```python
from build123d import *

# Parameters (mm, degrees)
SKETCH4_W           = 110
SKETCH4_H           = 80
BOSS_EXTRUDE1_DEPTH = 20
SHELL1_T            = -5
FILLET1_R           = 5
SKETCH8_W           = 15
SKETCH8_H           = 15
CUT_EXTRUDE2_DEPTH  = 5
SKETCH10_R          = 2
SKETCH10_R_2        = 1
BOSS_EXTRUDE2_DEPTH = 15
FILLET2_R           = 1


with BuildPart() as part:
    # Sketch4 → Boss-Extrude1 (new body)
    with BuildSketch(Plane(origin=(0, 0, 0), x_dir=(1, 0, 0), z_dir=(0, 1, 0))):
        Rectangle(SKETCH4_W, SKETCH4_H)
    extrude(amount=BOSS_EXTRUDE1_DEPTH)

    # Shell1
    shell1_openings = [part.faces().sort_by_distance(p)[0] for p in [
        (0, 20, 0),
    ]]
    offset(amount=SHELL1_T, openings=shell1_openings, kind=Kind.INTERSECTION)

    # Fillet1
    fillet1_edges = [part.edges().sort_by_distance(p)[0] for p in [
        (55, 10, 40),
        (-55, 10, 40),
        (-55, 10, -40),
        (55, 10, -40),
    ]]
    fillet(fillet1_edges, radius=FILLET1_R)

    # Sketch8 → Cut-Extrude2 (cut)
    with BuildSketch(Plane.ZY.offset(55)):
        with Locations((0, 12.5)):
            Rectangle(SKETCH8_W, SKETCH8_H)
    extrude(amount=-CUT_EXTRUDE2_DEPTH, mode=Mode.SUBTRACT)

    # Sketch10 → Boss-Extrude2 (add)
    # profile 1 of 4: a face of its own
    with BuildSketch(Plane(origin=(0, 5, 0), x_dir=(1, 0, 0), z_dir=(0, 1, 0))):
        with Locations(Location((47.1, 31.5, 0), (0, 0, 90))):
            Circle(SKETCH10_R)
        with Locations(Location((47.1, 31.5, 0), (0, 0, 90))):
            Circle(SKETCH10_R_2, mode=Mode.SUBTRACT)
    # profile 2 of 4: a face of its own
    with BuildSketch(Plane(origin=(0, 5, 0), x_dir=(1, 0, 0), z_dir=(0, 1, 0))):
        with Locations(Location((47.1, -31.5, 0), (0, 0, 90))):
            Circle(SKETCH10_R)
        with Locations(Location((47.1, -31.5, 0), (0, 0, 90))):
            Circle(SKETCH10_R_2, mode=Mode.SUBTRACT)
    # profile 3 of 4: a face of its own
    with BuildSketch(Plane(origin=(0, 5, 0), x_dir=(1, 0, 0), z_dir=(0, 1, 0))):
        with Locations(Location((-46.5, 31.5, 0), (0, 0, 90))):
            Circle(SKETCH10_R)
        with Locations(Location((-46.412417336, 31.528728885, 0), (0, 0, 90))):
            Circle(SKETCH10_R_2, mode=Mode.SUBTRACT)
    # profile 4 of 4: a face of its own
    with BuildSketch(Plane(origin=(0, 5, 0), x_dir=(1, 0, 0), z_dir=(0, 1, 0))):
        with Locations(Location((-46.5, -31.5, 0), (0, 0, 90))):
            Circle(SKETCH10_R)
        with Locations(Location((-46.412417336, -31.528728885, 0), (0, 0, 90))):
            Circle(SKETCH10_R_2, mode=Mode.SUBTRACT)
    extrude(amount=BOSS_EXTRUDE2_DEPTH)

    # Fillet2
    fillet2_edges = [part.edges().sort_by_distance(p)[0] for p in [
        (-55, 0, 0),
        (55, 0, 0),
        (0, 0, 40),
        (0, 0, -40),
        (-53.535533906, 0, 38.535533906),
        (53.535533906, 0, 38.535533906),
        (53.535533906, 0, -38.535533906),
        (-53.535533906, 0, -38.535533906),
    ]]
    fillet(fillet2_edges, radius=FILLET2_R)


solid = part.part
```
Source: CAD feature listing. Evaluate the final solid. Frame: model axes, mm. A direction names the side the tool comes from. Coordinates: 2 decimals unless noted, no trailing zeros. Write each loop counter-clockwise with the first axis right and the second up, starting at its lowest first coordinate (ties: lowest second). Pieces come first, ordered by that corner, then holes. Notation, with made-up numbers: (33, 82) - (58, 82) arc R19 cw to (58, 98) - close; hole circle Ø7 at (70.25, 32). An arc over 180 degrees is marked (long way). Answer as a JSON object with one key per item and string values.
Q1. Draft query along X for faces 4 (the cylindrical face through (48.874, 12.395, -32.423)), 5 (the cylindrical face through (-54, 11, 38)), 6 (the flat face through (-53, 12, -7.5)). Return one class per face: released by +X, released by -X, zero draft, split by the parting line, or undercut.
Ans:
{"face 4": "undercut", "face 5": "released by -X", "face 6": "zero draft"}
Q2. First-contact query: pin 1 Ø4 at (x, z) = (-23.5, -23) entering from +Y; pin 2 Ø2.5 at (x, y) = (-51.5, 11) entering from +Z; pin 3 Ø2.5 at (x, y) = (-53, 12.5) entering from -Z. Flat tips, straight axial feed; report the tip coordinate or a pass-through.
Ans:
{"pin 1": "stops at y = 5", "pin 2": "stops at z = 39.99", "pin 3": "stops at z = -39.68"}
Q3. Section query B-B, the plane z = 10. Output: boundary loops of the cut face in (x, y).
Ans:
{"outline": "(-55, 1) arc R1 ccw to (-54, 0) - (54, 0) arc R1 ccw to (55, 1) - (55, 20) - (50, 20) - (50, 5) - (-50, 5) - (-50, 20) - (-55, 20) - close"}
Q4. Set-up query: faces 1 (the flat face through (-1, 10, -40)), 2 (the flat face through (-53, 12, 7.5)), 3 (the cylindrical face through (48.874, 12.395, 30.577)). Return all of +Z, -Z, +X, -X, +Y, -Y with unobstructed straight access to the full face (end or side cutting, diameter ignored); none if empty.
Ans:
{"face 1": "-Z, +X, -X, +Y, -Y", "face 2": "-X, +Y", "face 3": "+Y"}
Q5. Material intervals for line 1 (Z direction, x = 47.1, y = 8.75); line 2 (X direction, y = 12.5, z = 31.5); line 3 (X direction, y = 8.5, z = 10), sorted ascending. Write a range as [from, to].
Ans:
{"line 1": "z = [-40, -35], [-33.5, -32.5], [-30.5, -29.5], [29.5, 30.5], [32.5, 33.5], [35, 40]", "line 2": "x = [-55, -50], [-48.5, -47.41], [-45.41, -44.5], [45.1, 46.1], [48.1, 49.1], [50, 55]", "line 3": "x = [-55, -50], [50, 55]"}
Q6. Section query C-C, the plane x = -28. Output: boundary loops of the cut face in (y, z).
Ans:
{"outline": "(0, -39) arc R1 ccw to (1, -40) - (20, -40) - (20, -35) - (5, -35) - (5, 35) - (20, 35) - (20, 40) - (1, 40) arc R1 ccw to (0, 39) - close"}
Q7. Section query A-A, the plane y = 13.5. State how many separate pieces and enclosed holes the cut face has, plus the area to 3 significant figures.
Ans:
{"separate pieces": "5", "enclosed holes": "4", "area": "1,740 mm2"}
